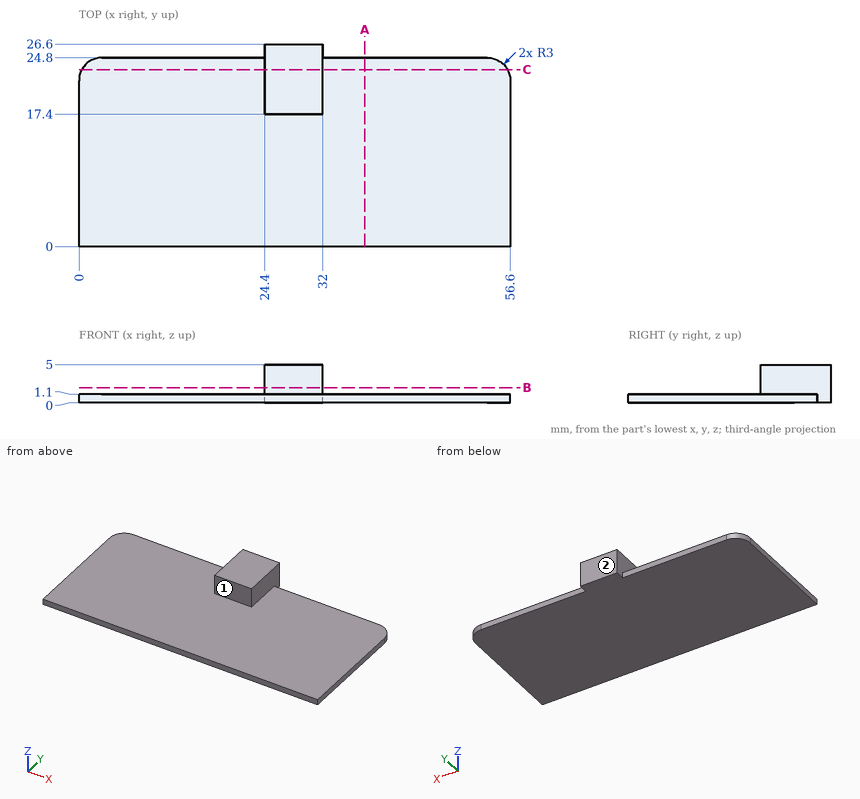
Here's the drawing with two shaded views (mm, measured from the low corner). I have some questions. A direction names the side the tool comes from. Give positions to 0.01 mm unless a question says otherwise; leave off trailing zeros. Loops run counter-clockwise (first coordinate to the right, second up) from the corner with the lowest first, then second, coordinate; pieces in that order, holes last. Notation, with made-up numbers: (26, -17.5) - (78, -17.5) arc R17 ccw to (78, -1.5) - close; hole circle Ø6 at (6.25, 78.25). An arc over 180 degrees is marked (long way). One line per item, written item: value.
(1) I'm going to push flat-ended pins straight in: pin 1 (0.6 mm diameter, centred on x = 40.5, z = 0.5, fed in from +Y); pin 2 (2 mm diameter, centred on x = 37, z = 3.5, fed in from -Y). Where does each tip first touch, or does it pass through?
Verdict:
pin 1: y = 24.8
pin 2: through
(2) If we section it at B-B, the plane z = 2: List the corners of the cut face in (x, y) for me, plus the area to 3 significant figures.
Verdict:
outline: (24.4, 17.4) - (32, 17.4) - (32, 26.6) - (24.4, 26.6) - close
area: 69.9 mm^2
(3) I need wall thicknesses on line 1 along Z through (x, y) = (33.5, 4); line 2 along Y through (x, z) = (22, 0.35); line 3 along X through (y, z) = (23.5, 1.85). Which ranges of each line are inside material? Lowest first, please.
Verdict:
line 1: 0 to 1.1
line 2: 0 to 24.8
line 3: 24.4 to 32
(4) On a 3-axis mill with a long thin cutter (end or side, diameter ignored), from which of +Z, -Z, +X, -X, +Y, -Y can I reach the whole of each face in a straight line? I mean the marked faces 1 and 2. Say none if no direction works.
Verdict:
face 1: +Z, +X, -X, -Y
face 2: +Z, -Z, +X, -X, +Y
(5) If we section it at A-A, the plane x = 37.5: List the corners of the cut face in (y, z) for me, plus the area to 3 significant figures.
Verdict:
outline: (0, 0) - (24.8, 0) - (24.8, 1.1) - (0, 1.1) - close
area: 27.3 mm^2
(6) If we section it at C-C, the plane y = 23.25: List the corners of the cut face in (x, z) for me, plus the area to 3 significant figures.
Verdict:
outline: (0.37, 0) - (56.23, 0) - (56.23, 1.1) - (32, 1.1) - (32, 5) - (24.4, 5) - (24.4, 1.1) - (0.37, 1.1) - close
area: 91.1 mm^2
